Can you work these out from the model? Positions are in its coordinate system, mm. Round coordinates to 2 decimals unless told otherwise and drop trailing zeros. Order: outer loops, then holes, each group sorted by start corner. A loop starts at its lowest first (then second) coordinate and runs counter-clockwise, first axis right, second up. Notation, with made-up numbers: M 60.25,35 L 66.25,35 A7 cw 66.25,45 Z; hole C -40,-29.5 d10. An arc over 180 degrees is marked long. Answer as a JSON object with one key per item and string values. Group by question number.
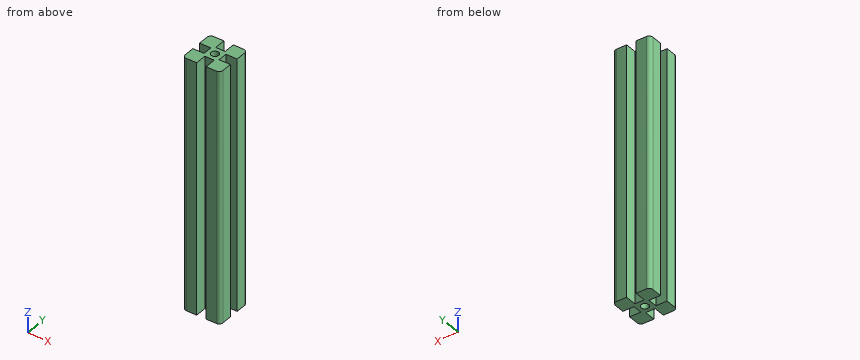
from build123d import *

# Parameters (mm, degrees)
F0_R     = 2
F1_DEPTH = 134
F2_R     = 2


with BuildPart() as f1:
    # F0 (on Top) → F1 (new body)
    with BuildSketch(Plane.XY):
        Polygon((-4, 2.5), (-4, 0), (-4, -2.5), (-10, -2.5), (-10, -10), (-2.5, -10), (-2.5, -4), (0, -4), (2.5, -4), (2.5, -10), (10, -10), (10, -2.5), (4, -2.5), (4, 0), (4, 2.5), (10, 2.5), (10, 10), (2.5, 10), (2.5, 4), (0, 4), (-2.5, 4), (-2.5, 10), (-10, 10), (-10, 2.5), align=None)
        Circle(F0_R, mode=Mode.SUBTRACT)
    extrude(amount=F1_DEPTH)

    # F2
    f2_edges = [f1.edges().sort_by_distance(p)[0] for p in [
        (10, -10, 67),
        (-10, -10, 67),
        (-10, 10, 67),
        (10, 10, 67),
    ]]
    fillet(f2_edges, radius=F2_R)


solid = f1.part
Item 1: I'm going to push flat-ended pins straight in: pin 1 Ø5 at (x, y) = (0, 0) entering from -Z; pin 2 Ø1.5 at (y, z) = (0.5, 67) entering from -X; pin 3 Ø2.5 at (y, z) = (0.5, 82.5) entering from +X. Where does each tip first touch, or does it pass through?
Item 2: Suppose I cut it at B-B, the plane y = 6. Write out the boundary of the cut face in (x, z), and give its area (3 significant figures).
Item 3: Suppose I cut it at C-C, the plane z = 43.5. Write out the boundary of the cut face in (x, y).
Item 4: Suppose I cut it at A-A, the plane x = 0. Write out the boundary of the cut face in (y, z).
Item 5: I need wall thicknesses on line 1 (Y direction, x = -6.5, z = 39.5); line 2 (Y direction, x = 0, z = 102.5). Which ranges of each line are inside material? Lowest first, please.
Computed:
{
 "1": {"pin 1": "stops at z = 0", "pin 2": "stops at x = -4", "pin 3": "stops at x = 4"},
 "2": {"outline": "M -10,0 L -2.5,0 L -2.5,134 L -10,134 Z; M 2.5,0 L 10,0 L 10,134 L 2.5,134 Z", "area": "2,010 mm^2"},
 "3": {"outline": "M -10,-8 A2 ccw -8,-10 L -2.5,-10 L -2.5,-4 L 2.5,-4 L 2.5,-10 L 8,-10 A2 ccw 10,-8 L 10,-2.5 L 4,-2.5 L 4,2.5 L 10,2.5 L 10,8 A2 ccw 8,10 L 2.5,10 L 2.5,4 L -2.5,4 L -2.5,10 L -8,10 A2 ccw -10,8 L -10,2.5 L -4,2.5 L -4,-2.5 L -10,-2.5 Z; hole C 0,0 d4"},
 "4": {"outline": "M -4,0 L -2,0 L -2,134 L -4,134 Z; M 2,0 L 4,0 L 4,134 L 2,134 Z"},
 "5": {"line 1": "y = -10 to -2.5, 2.5 to 10", "line 2": "y = -4 to -2, 2 to 4"}
}
